Verification items for the finished model (mm, model axes). A direction names the side the tool comes from. Coordinates: 2 decimals unless noted, no trailing zeros. Order: outer loops, then holes, each group sorted by start corner. A loop starts at its lowest first (then second) coordinate and runs counter-clockwise, first axis right, second up. Notation, with made-up numbers: M 33,68.25 L 77,68.25 A35 ccw 77,104.25 Z; hole C 17.5,53 d5. An arc over 180 degrees is marked long. Write item = value, one per line.
```python
from build123d import *

# Parameters (mm, degrees)
PAD_DEPTH    = 3
PAD001_DEPTH = 13
SKETCH001_W  = 4
SKETCH001_H  = 3
PAD002_DEPTH = 12
PAD003_DEPTH = 7
SKETCH005_R  = 2
PAD004_DEPTH = 2
FILLET_R     = 1.8
FILLET001_R  = 0.5
FILLET002_R  = 0.8


with BuildPart() as part:
    # Sketch → Pad (new body)
    with BuildSketch(Plane.XY):
        with BuildLine():
            Line((0, 0), (34, 0))
            Line((34, 0), (34, 8.5))
            Line((34, 8.5), (41, 35.5))
            ThreePointArc((41, 35.5), (26, 40.5), (11, 35.5))
            Line((16, 15), (11, 35.5))
            Line((4, 15), (16, 15))
            ThreePointArc((4, 15), (1.171573, 13.828427), (0, 11))
            Line((0, 0), (0, 11))
        make_face()
    extrude(amount=PAD_DEPTH)

    # Sketch002 → Pad001 (join)
    with BuildSketch(Plane.XY):
        Polygon((30.957764, 16.688984), (34.094791, 28.788945), (33.126794, 29.039907), (32.62487, 27.103913), (27.784885, 28.358724), (27.533923, 27.390727), (32.373908, 26.135916), (29.989767, 16.939946), align=None)
    extrude(amount=PAD001_DEPTH)

    # Sketch001 → Pad002 (join)
    with BuildSketch(Plane.XY):
        with Locations((13.5, 6)):
            Rectangle(SKETCH001_W, SKETCH001_H)
    extrude(amount=PAD002_DEPTH)

    # Sketch003 → Pad003 (join)
    with BuildSketch(Plane.XY):
        Polygon((34, 0), (34, 8.5), (38.485316, 25.800504), (37.517319, 26.051466), (33, 8.627522), (33, 0), align=None)
    extrude(amount=PAD003_DEPTH)

    # Sketch005 (on Face19 of Pad003) → Pad004 (join)
    with BuildSketch(Plane.XZ.offset(-4.5)):
        with Locations((13.490876, 10.002978)):
            Circle(SKETCH005_R)
    extrude(amount=PAD004_DEPTH)

    # Fillet
    fillet_edges = [part.edges().sort_by_distance(p)[0] for p in [
        (11.5, 6, 12),
        (15.5, 6, 12),
    ]]
    fillet(fillet_edges, radius=FILLET_R)

    # Fillet001
    fillet001_edges = [part.edges().sort_by_distance(p)[0] for p in [
        (11.490876, 2.5, 10.002978),
    ]]
    fillet(fillet001_edges, radius=FILLET001_R)

    # Fillet002
    fillet002_edges = [part.edges().sort_by_distance(p)[0] for p in [
        (36.242658, 17.150252, 0),
        (34, 4.25, 0),
        (33.5, 0, 0),
        (16.5, 0, 0),
        (0, 5.5, 0),
        (1.171573, 13.828427, 0),
        (10, 15, 0),
        (13.5, 25.25, 0),
        (26, 40.5, 0),
        (39.742658, 30.650252, 0),
    ]]
    fillet(fillet002_edges, radius=FILLET002_R)


solid = part.part
```
Item 1: Gauge pin test, flat ends, axial feed: pin 1 (2 mm diameter, centred on x = 14, z = 8.5, fed in from +Y); pin 2 (4 mm diameter, centred on x = 33.5, y = 26, fed in from +Z); pin 3 (1.1 mm diameter, centred on x = 11.5, z = 2, fed in from +Y); pin 4 (1 mm diameter, centred on y = 22, z = 8, fed in from -X). Record the tip position at first contact, or that the pin passes through.
Report:
pin_1 = 7.5
pin_2 = 13
pin_3 = 36.25
pin_4 = 31.17
Item 2: Release check for a two-part mould opening along X. For faces 1 (the flat face through (32.88, 28.09, 7.93)), 2 (the flat face through (13, 7.5, 7)), 3 (the cylindrical face through (13.806, 24.96, 0.241)) record: pulls with the +X half, pulls with the -X half, needs draft (parallel to the pull), parting line crosses it, or undercut.
Report:
face_1 = undercut
face_2 = needs draft
face_3 = pulls with the -X half
Item 3: Scan lines: L1, parallel to Z at x = 22.5, y = 15.5; L2, parallel to Y at x = 14, z = 7.75; L3, parallel to X at y = 6.5, z = 8. Record each from-to range of solid material in increasing order. Write a range as from..to.
Report:
L1 = 0..3
L2 = 4.5..7.5
L3 = 11.5..15.5
Item 4: Sectioned sample at B-B, the plane x = 5.5. Enter the section's corners in (y, z).
Report:
outline = M 0,0.8 A0.8 ccw 0.8,0 L 14.2,0 A0.8 ccw 15,0.8 L 15,3 L 0,3 Z
Item 5: Sectioned sample at A-A, the plane y = 3.5. Enter the section's corners in (x, z).
Report:
outline = M 0,0.8 A0.8 ccw 0.8,0 L 33.2,0 A0.8 ccw 34,0.8 L 34,7 L 33,7 L 33,3 L 0,3 Z; C 13.49,10 d4
Item 6: Tool access check on faces 4 (the flat face through (29.92, 26.772, 7.93)), 5 (the flat face through (27.66, 27.88, 7.93)), 6 (the flat face through (33, 4, 5)). Record the directions out of +Z, -Z, +X, -X, +Y, -Y that give a thin tool (end or side, any length) a straight path to the whole face; none if there is none.
Report:
face_4 = +Z, -X
face_5 = +Z, -X, +Y
face_6 = +Z, -Y
